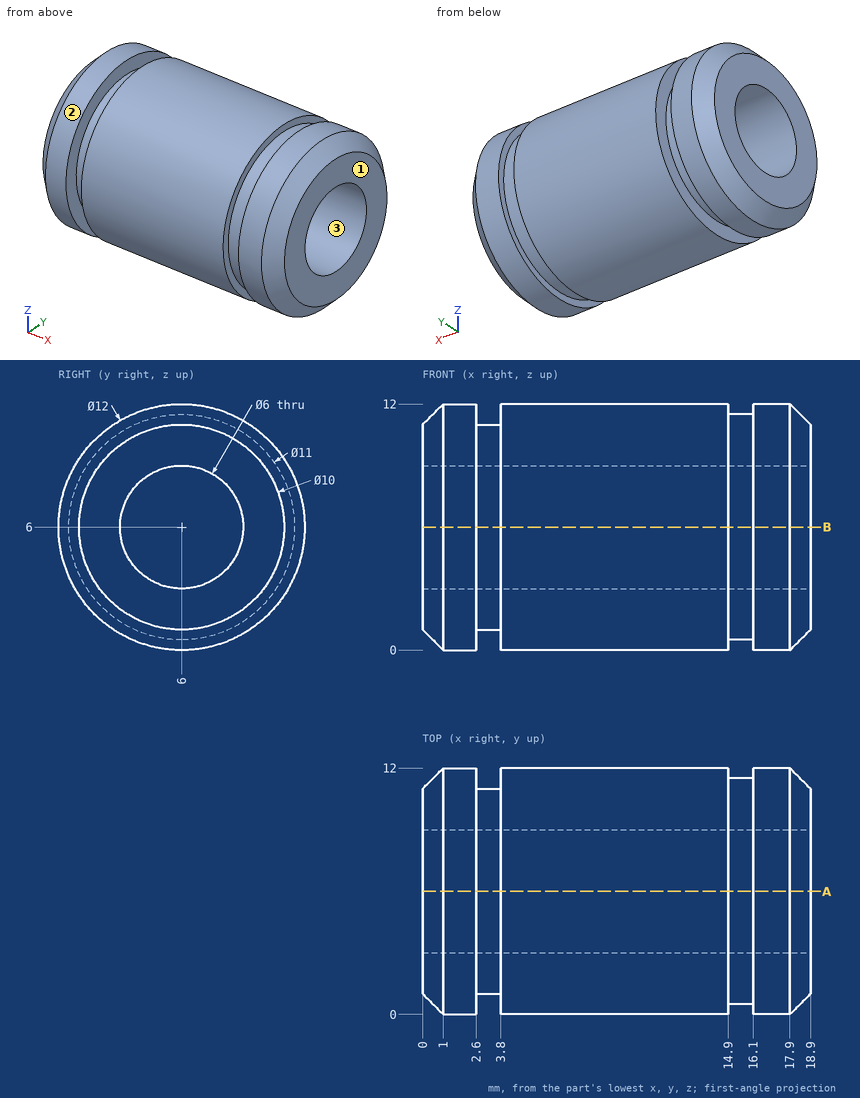
Part print with two shaded views. Sizes in mm from the minimum x, y, z corner. Give positions to 0.01 mm unless a question says otherwise; leave off trailing zeros. Write each loop counter-clockwise with the first axis right and the second up, starting at its lowest first coordinate (ties: lowest second). Pieces come first, ordered by that corner, then holes.
1) Probe L1, parallel to Y at x = 12, z = 6; L2, parallel to Y at x = 15, z = 6. List the from-to ranges inside material, lowest first.
Resolved:
L1: y = 0 to 3, 9 to 12
L2: y = 0.5 to 3, 9 to 11.5
2) Two-plate mould, pull along Y, no slides. Class the marked faces 1, 2 and 3: released by +Y, released by -Y, zero draft, split by the parting line, or undercut.
Resolved:
face 1: zero draft
face 2: split by the parting line
face 3: undercut
3) Pin check, flat tips, straight feed: pin 1 (5 mm diameter, centred on x = 10, y = 9, fed in from -Z); pin 2 (5 mm diameter, centred on y = 6, z = 6, fed in from -X); pin 3 (4 mm diameter, centred on x = 3.5, z = 2.5, fed in from +Y); pin 4 (1 mm diameter, centred on x = 3.5, y = 9, fed in from +Z). Stop position of each tip, or through.
Resolved:
pin 1: stops at z = 0.02
pin 2: passes through
pin 3: stops at y = 11.8
pin 4: stops at z = 11.41
4) Cut at A-A on y = 6. Write the cut outline in (x, z), then the cut area to 3 significant figures.
Resolved:
outline: (0, 1) - (1, 0) - (2.6, 0) - (2.6, 1) - (3.8, 1) - (3.8, 0) - (14.9, 0) - (14.9, 0.5) - (16.1, 0.5) - (16.1, 0) - (17.9, 0) - (18.9, 1) - (18.9, 3) - (0, 3) - close; (0, 9) - (18.9, 9) - (18.9, 11) - (17.9, 12) - (16.1, 12) - (16.1, 11.5) - (14.9, 11.5) - (14.9, 12) - (3.8, 12) - (3.8, 11) - (2.6, 11) - (2.6, 12) - (1, 12) - (0, 11) - close
area: 108 mm2
